Autodesk Inventor part; units mm, degrees
ref_plane "YZ Plane" through (0, 0, 0) normal (1, 0, 0) x (0, 1, 0)
ref_plane "XZ Plane" through (0, 0, 0) normal (0, 1, 0) x (-1, 0, 0)
ref_plane "XY Plane" through (0, 0, 0) normal (0, 0, 1) x (1, 0, 0)
sketch "Sketch1" plane through (0, 0, 0) normal (1, 0, 0) x (0, 1, 0)
  line L0 (22.0204, 54.3207) -> (-9.7296, 54.3207)
  line L1 (-9.7296, -34.5793) -> (22.0204, -34.5793)
  line L2 (22.0204, -34.5793) -> (22.0204, 54.3207)
  line L3 (15.6704, 44.7957) -> (-9.7296, 44.7957)
  line L4 (-9.7296, -25.0543) -> (15.6704, -25.0543)
  line L5 (15.6704, -25.0543) -> (15.6704, 44.7957)
  line L6 (-9.7296, 54.3207) -> (-9.7296, 44.7957)
  line L7 (-9.7296, -25.0543) -> (-9.7296, -34.5793)
  dimension "d0" = 88.9
  dimension "d2" = 6.35
  dimension "d3" = 9.525
  dimension "d4" = 9.525
  dimension "d7" = 25.4
  dimension "d8" = 0
extrude "Extrusion1" add sketch "Sketch1" along normal blind 9.525
sketch "Sketch2" plane through (0, 22.0204, 54.3207) normal (0, 1, 0) x (1, 0, 0)
  line L0 (0, 88.9) -> (9.525, 88.9)
  line L1 (0, 0) -> (9.525, 0)
  line L2 (0, 88.9) -> (0, 0)
  point P0 (0, 54.3207)
  point P1 (4.7625, 5.08)
  point P2 (4.7625, 83.82)
  dimension "d9" = 5.08
  dimension "d10" = 5.08
  dimension "d11" = 4.7625
  dimension "d12" = 0
hole "Hole1" at (4.7625, 22.0204, 49.2407) at (4.7625, 22.0204, -29.4993) direction (0, -1, 0) diameter 4.4958 end through all
sketch "Sketch4" plane through (0, 0, 0) normal (-1, 0, 0) x (0, 0, 1)
  line L0 (44.7957, 15.6704) -> (-25.0543, 15.6704)
  line L1 (44.7957, -9.7296) -> (44.7957, 15.6704)
  line L2 (-25.0543, 15.6704) -> (-25.0543, -9.7296)
  line L3 (-25.0543, 10.5904) -> (-19.9743, 15.6704)
  line L4 (-19.9743, 15.6704) -> (-25.0543, 15.6704)
  line L5 (-25.0543, 15.6704) -> (-25.0543, 10.5904)
  line L6 (44.7957, 10.5904) -> (44.7957, 15.6704)
  line L7 (44.7957, 15.6704) -> (39.7157, 15.6704)
  line L8 (39.7157, 15.6704) -> (44.7957, 10.5904)
  point P0 (0, 0)
  dimension "d20" = 45
  dimension "d21" = 5.08
  dimension "d22" = 0
  dimension "d23" = 0
  dimension "d24" = 45
  dimension "d25" = 5.08
  dimension "d26" = 0
  dimension "d27" = 0
extrude "Extrusion2" add sketch "Sketch4" against normal blind 5
sketch "Sketch5" plane through (0, 0, 0) normal (-1, 0, 0) x (0, 0, 1)
  line L0 (7.0767, 15.6704) -> (12.6647, 15.6704)
  line L1 (12.6647, 15.6704) -> (9.8707, 12.8764)
  line L2 (9.8707, 12.8764) -> (7.0767, 15.6704)
  line L3 (39.7157, 15.6704) -> (-19.9743, 15.6704)
  line L4 (-34.5793, -9.7296) -> (-34.5793, 22.0204)
  point P0 (0, 0)
  dimension "d30" = 90
  dimension "d31" = 45
  dimension "d32" = 2.794
  dimension "d33" = 0
  dimension "d34" = 44.45
extrude "Extrusion3" add sketch "Sketch5" against normal blind 5
sketch "Sketch6" plane through (0, 0, 0) normal (-1, 0, 0) x (0, 0, 1)
  line L0 (-0.2893, 9.5064) -> (-15.5293, 9.5064)
  line L1 (-15.5293, 9.5064) -> (-15.5293, 17.7024)
  line L2 (-15.5293, 17.7024) -> (-0.2893, 17.7024)
  line L3 (-0.2893, 17.7024) -> (-0.2893, 9.5064)
  line L4 (35.2707, 11.3259) -> (20.0307, 11.3259)
  line L5 (20.0307, 11.3259) -> (20.0307, 17.7024)
  line L6 (20.0307, 17.7024) -> (35.2707, 17.7024)
  line L7 (35.2707, 17.7024) -> (35.2707, 11.3259)
  line L8 (39.7157, 15.6704) -> (12.6647, 15.6704)
  line L9 (-34.5793, -9.7296) -> (-34.5793, 22.0204)
  line L10 (54.3207, 22.0204) -> (54.3207, -9.7296)
  point P0 (0, 0)
  dimension "d37" = 2.032
  dimension "d38" = 0
  dimension "d39" = 19.05
  dimension "d40" = 19.05
  dimension "d42" = 15.24
  dimension "d43" = 15.24
extrude "Extrusion4" cut sketch "Sketch6" against normal blind 254
properties part number "SparkMaxTop"
Geometry: final body of the model. Coordinates: model frame, mm. A direction names the side the tool comes from. Coordinates: 2 decimals unless noted, no trailing zeros. Order: outer loops, then holes, each group sorted by start corner. A loop starts at its lowest first (then second) coordinate and runs counter-clockwise, first axis right, second up.
(1) Section query D-D (x = 8). Return the cut outline in (y, z).
(2) First-contact query: pin 1 (5 mm diameter, centred on x = 3, z = 41, fed in from -Y); pin 2 (5 mm diameter, centred on x = 4, z = -19.5, fed in from -Y); pin 3 (2 mm diameter, centred on y = 14.5, z = 10.5, fed in from +X). Flat tips, straight axial feed; report the tip coordinate or a pass-through.
(3) Section query A-A (y = 14). Return the cut outline in (x, z) (1 decimal).
(4) Draft query along Z for faces 1 (the face through (5, -9.73, 52)), 2 (the face through (5, 17, -0.289)). Return one class per face: pulls with the +Z half, pulls with the -Z half, needs draft (parallel to the pull), parting line crosses it, or undercut.
(5) Access query for faces 3 (the face through (6, 15.67, 39)), 4 (the face through (5.62, 5.92, 51.32)), 5 (the face through (5, 17, -15.529)). Directions: +Z, -Z, +X, -X, +Y, -Y. A direction counts if a zero-diameter tool reaches every point of the face in a straight line with its end or side. Return the directions, or none.
(6) Material intervals for probe 1 along Z at (x, y) = (7.5, 16.5); probe 2 along Z at (x, y) = (4.75, -4.5); probe 3 along Z at (x, y) = (8.25, 4), sorted ascending.
(7) Section query B-B (x = 4). State how many separate pieces and enclosed holes the cut face has, plus the area to 3 significant figures.
(8) Section query C-C (y = 2.5). Return the cut outline in (x, z) (1 decimal), plus the area to 3 significant figures.
Solution:
1. outline: (-9.73, -34.58) - (22.02, -34.58) - (22.02, 54.32) - (-9.73, 54.32) - (-9.73, 44.8) - (15.67, 44.8) - (15.67, 35.27) - (17.7, 35.27) - (17.7, 20.03) - (15.67, 20.03) - (15.67, -0.29) - (17.7, -0.29) - (17.7, -15.53) - (15.67, -15.53) - (15.67, -25.05) - (-9.73, -25.05) - close
2. pin 1: stops at y = 11.89
2. pin 2: stops at y = 13.64
2. pin 3: stops at x = 5
3. outline: (0, -34.6) - (9.5, -34.6) - (9.5, -25.1) - (5, -25.1) - (5, -21.6) - (0, -21.6) - close; (0, 8.7) - (5, 8.7) - (5, 11) - (0, 11) - close; (0, 41.4) - (5, 41.4) - (5, 44.8) - (9.5, 44.8) - (9.5, 54.3) - (0, 54.3) - close; hole circle Ø4.5 at (4.8, -29.5); hole circle Ø4.5 at (4.8, 49.2)
4. face 1: needs draft
4. face 2: undercut
5. face 3: +X, -Y
5. face 4: +Y, -Y
5. face 5: +X, -X, -Y
6. probe 1: z = -34.58 to -15.53, -0.29 to 20.03, 35.27 to 54.32
6. probe 2: z = -34.58 to -31.75, -27.25 to -25.05, 44.8 to 46.99, 51.49 to 54.32
6. probe 3: z = -34.58 to -25.05, 44.8 to 54.32
7. separate pieces: 3
7. enclosed holes: 0
7. area: 752 mm2
8. outline: (0, -34.6) - (9.5, -34.6) - (9.5, -25.1) - (0, -25.1) - close; (0, 44.8) - (9.5, 44.8) - (9.5, 54.3) - (0, 54.3) - close; hole circle Ø4.5 at (4.8, -29.5); hole circle Ø4.5 at (4.8, 49.2)
8. area: 150 mm2
